Study the drawing (mm; zero at the part's minimum x, y, z) and answer. A direction names the side the tool comes from. Coordinates: 2 decimals unless noted, no trailing zeros. Order: outer loops, then holes, each group sorted by start corner. A loop starts at its lowest first (then second) coordinate and runs counter-clockwise, first axis right, second up. Notation, with made-up numbers: M 33.25,25 L 86.25,25 A15 cw 86.25,42 Z; hole C -16,71.25 d10. An arc over 180 degrees is marked long. Use a Markdown table: item, result. Add a question column.
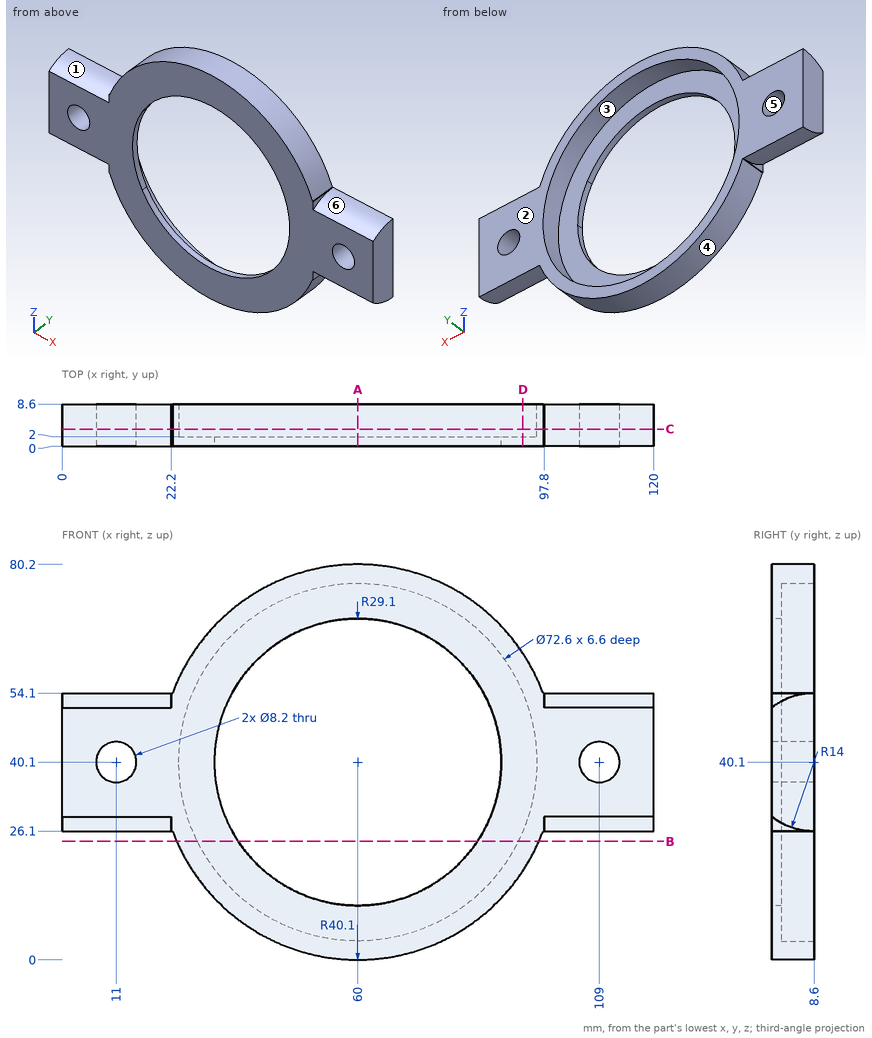
(1) Given P1, Ø1.5, axis at x = 92.5, y = 7.5, coming from the -Z side; P2, Ø4, axis at x = 54, y = 5, coming from the -Z side, each flat-ended and moving along its own axis, determine where each tip first touches the part or whether it passes through.
(2) Straight lines are drawn through the part: line 1 (Z direction, x = 60, y = 3.75); line 2 (X direction, y = 1.5, z = 43); line 3 (X direction, y = 7, z = 63.5). For each, find the intervals that lie inside material, in ascending order.
(3) A cutting plane is placed at B-B on z = 24. Write down the section's boundary in (x, y), plus the area to 3 significant figures.
(4) A cutting plane is placed at C-C on y = 3.5. Write down the section's boundary in (x, z), plus the area to 3 significant figures.
(5) A cutting plane is placed at A-A on x = 60. Write down the section's boundary in (y, z).
(6) The mould has two halves that part along Z. Classify the marked faces 4, 5 and 6: pulls with the +Z half, pulls with the -Z half, needs draft (parallel to the pull), parting line crosses it, or undercut.
(7) Which of the six approach directions +Z, -Z, +X, -X, +Y, -Y give full straight-line access (tool end or side, diameter ignored) to the marked faces 1, 2 and 3?
(8) A cutting plane is placed at D-D on x = 93.5. Write down the section's boundary in (y, z), plus the area to 3 significant figures.
From the geometry:
| question | item | result |
|---|---|---|
| 1 | P1 | stops at z = 15.61 |
| 1 | P2 | stops at z = 0.2 |
| 2 | line 1 | z = 0 to 3.8, 76.4 to 80.2 |
| 2 | line 2 | x = 0 to 8.1, 13.9 to 31.04, 88.96 to 106.1, 111.9 to 120 |
| 2 | line 3 | x = 27.44 to 32.25, 87.75 to 92.56 |
| 3 | outline | M 23.27,0 L 35.76,0 L 35.76,2 L 27.47,2 L 27.47,8.6 L 23.27,8.6 Z; M 84.24,0 L 96.73,0 L 96.73,8.6 L 92.53,8.6 L 92.53,2 L 84.24,2 Z |
| 3 | area | 105 mm2 |
| 4 | outline | M 0,27.06 L 22.2,27.06 L 22.2,26.1 L 22.42,26.1 A40.1 ccw 97.58,26.1 L 97.8,26.1 L 97.8,27.06 L 120,27.06 L 120,53.14 L 97.8,53.14 L 97.8,54.1 L 97.58,54.1 A40.1 ccw 22.42,54.1 L 22.2,54.1 L 22.2,53.14 L 0,53.14 Z; hole C 11,40.1 d8.2; hole C 60,40.1 d72.6; hole C 109,40.1 d8.2 |
| 4 | area | 1,880 mm2 |
| 5 | outline | M 0,0 L 8.6,0 L 8.6,3.8 L 2,3.8 L 2,11 L 0,11 Z; M 0,69.2 L 2,69.2 L 2,76.4 L 8.6,76.4 L 8.6,80.2 L 0,80.2 Z |
| 6 | face 4 | pulls with the -Z half |
| 6 | face 5 | undercut |
| 6 | face 6 | pulls with the +Z half |
| 7 | face 1 | +Z, -X, -Y |
| 7 | face 2 | +Z, -Z, +X, -X, +Y |
| 7 | face 3 | +Y |
| 8 | outline | M 0,18.06 L 8.6,18.06 L 8.6,26.12 L 2,26.12 L 2,54.08 L 8.6,54.08 L 8.6,62.14 L 0,62.14 Z |
| 8 | area | 195 mm2 |
